from build123d import *

# Parameters (mm, degrees)
SKETCH_1_W          = 50
SKETCH_1_H          = 70
EXTRUDE_1_DEPTH     = 28
CUT_EXTRUDE_6_DEPTH = 52.322509681
CHAMFER_1_SIZE      = 15
CHAMFER_1_SIZE2     = 2.644904711
CHAMFER_2_SIZE      = 15
CHAMFER_2_SIZE2     = 2.644904711
SKETCH_6_W          = 24
SKETCH_6_H          = 0.5
CUT_EXTRUDE_7_DEPTH = 80.429213769
SKETCH_7_W          = 0.5
SKETCH_7_H          = 12
CUT_EXTRUDE_8_DEPTH = 80.429213769
CHAMFER_3_SIZE      = 2


with BuildPart() as part:
    # 草圖1 → 伸長1 (new body)
    with BuildSketch(Plane.XY):
        Rectangle(SKETCH_1_W, SKETCH_1_H)
    extrude(amount=EXTRUDE_1_DEPTH)

    # 草圖4 → 除料-伸長6 (cut, through all)
    with BuildSketch(Plane.XY.offset(28)):
        with BuildLine():
            Line((-9.2, 35), (-9.2, 25))
            Line((-9.2, 25), (-13.5, 25))
            ThreePointArc((-13.5, 25), (-18.5, 20), (-13.5, 15))
            Line((-13.5, 15), (13.5, 15))
            ThreePointArc((13.5, 15), (18.5, 20), (13.5, 25))
            Line((13.5, 25), (9.2, 25))
            Line((9.2, 25), (9.2, 35))
            Line((9.2, 35), (-9.2, 35))
        make_face()
    extrude(amount=-CUT_EXTRUDE_6_DEPTH, mode=Mode.SUBTRACT)

    # 導角1
    chamfer_1_edges = [part.edges().sort_by_distance(p)[0] for p in [
        (0, -35, 0),
    ]]
    chamfer_1_side = [part.faces().sort_by_distance(p)[0] for p in [
        (0, -4.209254903, 0),
    ]]
    chamfer(chamfer_1_edges, length=CHAMFER_1_SIZE, length2=CHAMFER_1_SIZE2, reference=chamfer_1_side[0])

    # 導角2
    chamfer_2_edges = [part.edges().sort_by_distance(p)[0] for p in [
        (0, -35, 28),
    ]]
    chamfer_2_side = [part.faces().sort_by_distance(p)[0] for p in [
        (0, -4.209254903, 28),
    ]]
    chamfer(chamfer_2_edges, length=CHAMFER_2_SIZE, length2=CHAMFER_2_SIZE2, reference=chamfer_2_side[0])

    # 草圖6 → 除料-伸長7 (cut, through all)
    with BuildSketch(Plane(origin=(0, 35, 0), x_dir=(1, 0, 0), z_dir=(0, 1, 0))):
        with Locations((0, -27.75)):
            Rectangle(SKETCH_6_W, SKETCH_6_H)
        with Locations((0, -0.25)):
            Rectangle(SKETCH_6_W, SKETCH_6_H)
    extrude(amount=-CUT_EXTRUDE_7_DEPTH, mode=Mode.SUBTRACT)

    # 草圖7 → 除料-伸長8 (cut, through all)
    with BuildSketch(Plane(origin=(0, 35, 0), x_dir=(1, 0, 0), z_dir=(0, 1, 0))):
        with Locations((-24.75, -14)):
            Rectangle(SKETCH_7_W, SKETCH_7_H)
        with Locations((24.75, -14)):
            Rectangle(SKETCH_7_W, SKETCH_7_H)
    extrude(amount=-CUT_EXTRUDE_8_DEPTH, mode=Mode.SUBTRACT)

    # 導角3
    chamfer_3_edges = [part.edges().sort_by_distance(p)[0] for p in [
        (-25, 7.5, 28),
        (25, 7.5, 0),
        (25, 7.5, 28),
        (-25, 7.5, 0),
    ]]
    chamfer(chamfer_3_edges, length=CHAMFER_3_SIZE)


solid = part.part
Design review of the part built by this model. Coordinates are the model's own, in mm. A direction names the side the tool comes from. Round coordinates to 2 decimals unless told otherwise and drop trailing zeros. Write each loop counter-clockwise with the first axis right and the second up, starting at its lowest first coordinate (ties: lowest second). Pieces come first, ordered by that corner, then holes. Notation, with made-up numbers: (56.5, 7.25) -> (86.5, 7.25) arc R27 ccw to (86.5, 42.25) -> close; hole circle Ø10 at (-36, 60.25). An arc over 180 degrees is marked (long way). One line per item, written item: value. Start each with the question number.
Q1. Add section D-D (z = 23.5). Give the boundary of the cut face in (x, y), then the cut area to 3 significant figures.
Q2. To check wall thickness, follow probe 1 along Y at (x, z) = (11, 5.25); probe 2 along Y at (x, z) = (-5, 7.25); probe 3 along X at (y, z) = (6, 9.25). State the ranges of each line that lie inside material, in increasing order.
Q3. The part is to be moulded in two halves that separate along X. For faces 6 (the face through (-24, 1, 1)), 7 (the face through (25, 0, 23)), 8 (the face through (-18.5, 20.1, 14.2)), say which applies: pulls with the +X half, pulls with the -X half, needs draft (parallel to the pull), parting line crosses it, or undercut.
Q4. Add section A-A (y = 29). Give the boundary of the cut face in (x, z), then the cut area to 3 significant figures.
Q5. Add section C-C (y = 4.5). Give the boundary of the cut face in (x, z), then the cut area to 3 significant figures.
Q6. Insertion check: P1, Ø0.6, axis at y = 30, z = 27.5, coming from the +X side; P2, Ø3, axis at y = 23.5, z = 12, coming from the +X side; P3, Ø7, axis at x = -5, y = -2.5, coming from the +Z side. Each pin has a flat end and moves straight along its axis. Give the tip position at first contact, or say it passes through.
Q7. Add section B-B (x = 11). Give the boundary of the cut face in (y, z).
Q8. Tool access review of faces 1 (the face through (-11, 30, 0.5)), 2 (the face through (11, 30, 27.5)), 3 (the face through (-9.2, 30, 14)), 4 (the face through (11, 25, 14)), 5 (the face through (-24.5, 0, 14)): name each direction out of +Z, -Z, +X, -X, +Y, -Y from which nothing blocks a thin tool from reaching the whole face with its end or side.
Response:
1. outline: (-25, -35) -> (25, -35) -> (25, 35) -> (9.2, 35) -> (9.2, 25) -> (13.5, 25) arc R5 cw to (13.5, 15) -> (-13.5, 15) arc R5 cw to (-13.5, 25) -> (-9.2, 25) -> (-9.2, 35) -> (-25, 35) -> close
1. area: 2,970 mm^2
2. probe 1: y = -35 to 15, 25 to 35
2. probe 2: y = -35 to 15
2. probe 3: x = -24.5 to 24.5
3. face 6: pulls with the -X half
3. face 7: pulls with the +X half
3. face 8: undercut
4. outline: (-25, 2) -> (-23, 0) -> (-12, 0) -> (-12, 0.5) -> (-9.2, 0.5) -> (-9.2, 27.5) -> (-12, 27.5) -> (-12, 28) -> (-23, 28) -> (-25, 26) -> (-25, 20) -> (-24.5, 20) -> (-24.5, 8) -> (-25, 8) -> close; (9.2, 0.5) -> (12, 0.5) -> (12, 0) -> (23, 0) -> (25, 2) -> (25, 8) -> (24.5, 8) -> (24.5, 20) -> (25, 20) -> (25, 26) -> (23, 28) -> (12, 28) -> (12, 27.5) -> (9.2, 27.5) -> close
4. area: 859 mm^2
5. outline: (-25, 2) -> (-23, 0) -> (-12, 0) -> (-12, 0.5) -> (12, 0.5) -> (12, 0) -> (23, 0) -> (25, 2) -> (25, 8) -> (24.5, 8) -> (24.5, 20) -> (25, 20) -> (25, 26) -> (23, 28) -> (12, 28) -> (12, 27.5) -> (-12, 27.5) -> (-12, 28) -> (-23, 28) -> (-25, 26) -> (-25, 20) -> (-24.5, 20) -> (-24.5, 8) -> (-25, 8) -> close
5. area: 1,360 mm^2
6. P1: stops at x = 23.8
6. P2: stops at x = 24.5
6. P3: stops at z = 27.5
7. outline: (-35, 2.64) -> (-22.84, 0.5) -> (15, 0.5) -> (15, 27.5) -> (-22.84, 27.5) -> (-35, 25.36) -> close; (25, 0.5) -> (35, 0.5) -> (35, 27.5) -> (25, 27.5) -> close
8. face 1: -Z, +Y, -Y
8. face 2: +Z, +Y, -Y
8. face 3: +Z, -Z, +Y
8. face 4: +Z, -Z
8. face 5: -X, +Y, -Y
